Input: part model. Units: mm. Frame: model coordinates. Round coordinates to 2 decimals unless told otherwise and drop trailing zeros. Order: outer loops, then holes, each group sorted by start corner. A loop starts at its lowest first (then second) coordinate and runs counter-clockwise, first axis right, second up. Notation, with made-up numbers: (-13.5, 29) - (39.5, 29) arc R17 cw to (39.5, 58) - close; hole circle Ø5 at (-23.75, -5.5). An arc over 180 degrees is marked (long way). One line per item, written item: value. Start each with the question number.
from build123d import *

# Parameters (mm, degrees)
SKETCH1_W           = 208.8
SKETCH1_H           = 67.2
BOSS_EXTRUDE1_DEPTH = 25.4
FILLET1_R           = 10
SKETCH2_R           = 1.9
BOSS_EXTRUDE2_DEPTH = 5
SKETCH4_R           = 0.95
BOSS_EXTRUDE3_DEPTH = 3
SKETCH5_W           = 20
SKETCH5_H           = 50.8
BOSS_EXTRUDE4_DEPTH = 0.0001
BOSS_EXTRUDE5_DEPTH = 0.0001
BOSS_EXTRUDE6_DEPTH = 0.0001
FILLET7_R           = 1
FILLET8_R           = 1


with BuildPart() as part:
    # Sketch1 → Boss-Extrude1 (new, symmetric)
    with BuildSketch(Plane(origin=(0, 0, 0), x_dir=(1, 0, 0), z_dir=(0, 1, 0))):
        Rectangle(SKETCH1_W, SKETCH1_H)
    extrude(amount=BOSS_EXTRUDE1_DEPTH, both=True)

    # Fillet1
    fillet1_edges = [part.edges().sort_by_distance(p)[0] for p in [
        (-104.4, 25.4, 0),
        (-104.4, -25.4, 0),
    ]]
    fillet(fillet1_edges, radius=FILLET1_R)

    # Sketch2 → Boss-Extrude2 (add)
    with BuildSketch(Plane(origin=(0, 0, -33.6), x_dir=(-1, 0, 0), z_dir=(0, 0, -1))):
        with Locations(Location((96.4, 3.35, 0), (0, 0, 180))):
            Circle(SKETCH2_R)
        with Locations(Location((96.4, -3.35, 0), (0, 0, 180))):
            Circle(SKETCH2_R)
    extrude(amount=BOSS_EXTRUDE2_DEPTH)

    # Sketch4 → Boss-Extrude3 (add)
    with BuildSketch(Plane.XY.offset(33.6)):
        with Locations(Location((-99.4, 3.3, 0), (0, 0, 180))):
            Circle(SKETCH4_R)
        with Locations(Location((-99.4, 1.1, 0), (0, 0, 180))):
            Circle(SKETCH4_R)
        with Locations(Location((-99.4, -1.1, 0), (0, 0, 180))):
            Circle(SKETCH4_R)
        with Locations(Location((-99.4, -3.3, 0), (0, 0, 180))):
            Circle(SKETCH4_R)
    extrude(amount=BOSS_EXTRUDE3_DEPTH)

    # Sketch5 → Boss-Extrude4 (add)
    with BuildSketch(Plane.XY.offset(33.6)):
        with Locations((-84.4, 0)):
            Rectangle(SKETCH5_W, SKETCH5_H)
    boss_extrude4 = extrude(amount=BOSS_EXTRUDE4_DEPTH)

    # Mirror1: Boss-Extrude4 across plane
    add(boss_extrude4.mirror(Plane.XY))

    # Mirror1 at the second plane: Boss-Extrude4 across plane
    add(boss_extrude4.mirror(Plane.ZX))

    # Sketch6 → Boss-Extrude5 (add)
    with BuildSketch(Plane(origin=(0, 25.4, 0), x_dir=(1, 0, 0), z_dir=(0, 1, 0))):
        with BuildLine():
            Line((16.9, 13.2), (92.7, 13.2))
            ThreePointArc((92.7, 13.2), (94.114213562, 12.614213562), (94.7, 11.2))
            Line((94.7, 11.2), (94.7, -11.2))
            ThreePointArc((94.7, -11.2), (94.114213562, -12.614213562), (92.7, -13.2))
            Line((92.7, -13.2), (16.9, -13.2))
            ThreePointArc((16.9, -13.2), (15.485786438, -12.614213562), (14.9, -11.2))
            Line((14.9, -11.2), (14.9, 11.2))
            ThreePointArc((14.9, 11.2), (15.485786438, 12.614213562), (16.9, 13.2))
        make_face()
    extrude(amount=BOSS_EXTRUDE5_DEPTH)

    # Sketch7 → Boss-Extrude6 (add)
    with BuildSketch(Plane.XZ.offset(25.4)):
        with BuildLine():
            Line((28.8, 12.5), (79.7, 12.5))
            ThreePointArc((79.7, 12.5), (81.114213562, 11.914213562), (81.7, 10.5))
            Line((81.7, 10.5), (81.7, -10.5))
            ThreePointArc((81.7, -10.5), (81.114213562, -11.914213562), (79.7, -12.5))
            Line((79.7, -12.5), (28.8, -12.5))
            ThreePointArc((28.8, -12.5), (27.385786438, -11.914213562), (26.8, -10.5))
            Line((26.8, -10.5), (26.8, 10.5))
            ThreePointArc((26.8, 10.5), (27.385786438, 11.914213562), (28.8, 12.5))
        make_face()
    extrude(amount=BOSS_EXTRUDE6_DEPTH)

    # Fillet7
    fillet7_edges = [part.edges().sort_by_distance(p)[0] for p in [
        (104.4, 25.4, 0),
        (-104.4, 0, 33.6),
        (-104.4, 0, -33.6),
        (15, 25.4, -33.6),
        (-101.471067812, 22.471067812, 33.6),
        (-101.471067812, -22.471067812, 33.6),
        (-101.471067812, 22.471067812, -33.6),
        (-101.471067812, -22.471067812, -33.6),
        (15, -25.4, -33.6),
        (104.4, -25.4, 0),
        (15, -25.4, 33.6),
        (15, 25.4, 33.6),
        (104.4, 0, -33.6),
        (104.4, 0, 33.6),
    ]]
    fillet(fillet7_edges, radius=FILLET7_R)

    # Fillet8
    fillet8_edges = [part.edges().sort_by_distance(p)[0] for p in [
        (-84.4, -25.4, 33.6001),
        (-84.4, 25.4, 33.6001),
        (-84.4, 25.4, -33.6001),
        (-84.4, -25.4, -33.6001),
    ]]
    fillet(fillet8_edges, radius=FILLET8_R)


solid = part.part
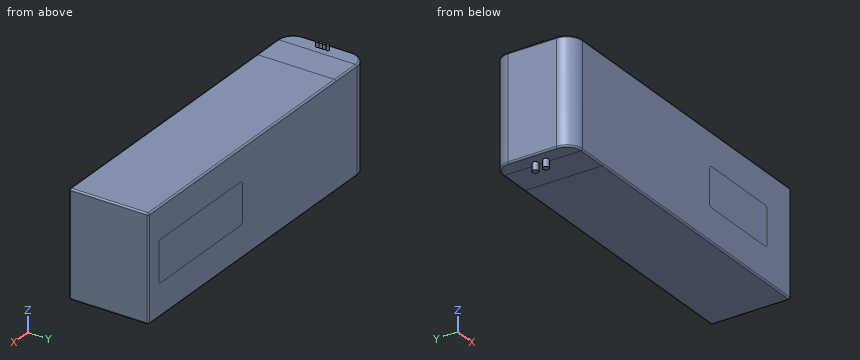
Item 1: First-contact query: pin 1 Ø4.5 at (x, y) = (-98.5, 9) entering from -Z; pin 2 Ø4 at (x, y) = (64, -6) entering from +Z. Flat tips, straight axial feed; report the tip coordinate or a pass-through.
Item 2: Section query C-C on x = -38.5. Return loops of the section in (y, z), and give its area (3 significant figures).
Item 3: Line query: L1, parallel to Z at x = 5, y = 21; L2, parallel to X at y = 23, z = 30.5; L3, parallel to X at y = -20, z = 27. Output: solid intervals per line, ascending.
Geometry results:
1. pin 1: stops at z = -33.6
1. pin 2: stops at z = 33.6
2. outline: (-25.4, -32.6) arc R1 ccw to (-24.4, -33.6) - (24.4, -33.6) arc R1 ccw to (25.4, -32.6) - (25.4, 32.6) arc R1 ccw to (24.4, 33.6) - (-24.4, 33.6) arc R1 ccw to (-25.4, 32.6) - close
2. area: 3,410 mm^2
3. L1: z = -33.6 to 33.6
3. L2: x = -100.9 to 104.4
3. L3: x = -103.28 to 104.4
